Check sheet for the drawn part. Datum: minimum x, y, z corner. Units: mm. A direction names the side the tool comes from. Round coordinates to 2 decimals unless told otherwise and drop trailing zeros. Write each loop counter-clockwise with the first axis right and the second up, starting at its lowest first coordinate (ties: lowest second). Pieces come first, ordered by that corner, then holes. Notation, with made-up numbers: (-24, 29.5) - (1, 29.5) arc R33 ccw to (1, 68.5) - close; hole circle Ø4 at (50, -38.5). An arc over 180 degrees is marked (long way). Answer as a JSON object with one key per item and string values. Group by question number.
1) Mould release check, pull along Z, two halves, no side actions. Record for the marked faces 3, 4 and 5: +Z half, -Z half, draft (parallel to the pull), parting line (faces both ways), or undercut.
2) Go/stop test with flat-tipped pins: pin 1 Ø2 at (x, y) = (8, 6) entering from -Z; pin 2 Ø1 at (x, y) = (10, 2) entering from +Z; pin 3 Ø8 at (y, z) = (8.5, 15.5) entering from +X; pin 4 Ø6.5 at (x, z) = (17.5, 5) entering from +Y. Record where each tip stops, or that it passes through.
3) Thickness scan on line 1 (Z direction, x = 17.5, y = 3.1); line 2 (Z direction, x = 17.5, y = 9.75). Record the ranges inside material, lowest first.
4) Set-up check for the marked faces 1 and 2: record each of +Z, -Z, +X, -X, +Y, -Y from which the full face is reachable in a straight line by a thin tool's end or side.
5) Section check A-A (x = 17.5). Enter the section's corners in (y, z).
6) Section check D-D (x = 12.5). Enter the section's corners in (y, z).
7) Section check B-B (z = 30). Enter the section's corners in (x, y), then the cut area to 3 significant figures.
8) Section check C-C (z = 17.5). Enter the section's corners in (x, y), then the cut area to 3 significant figures.
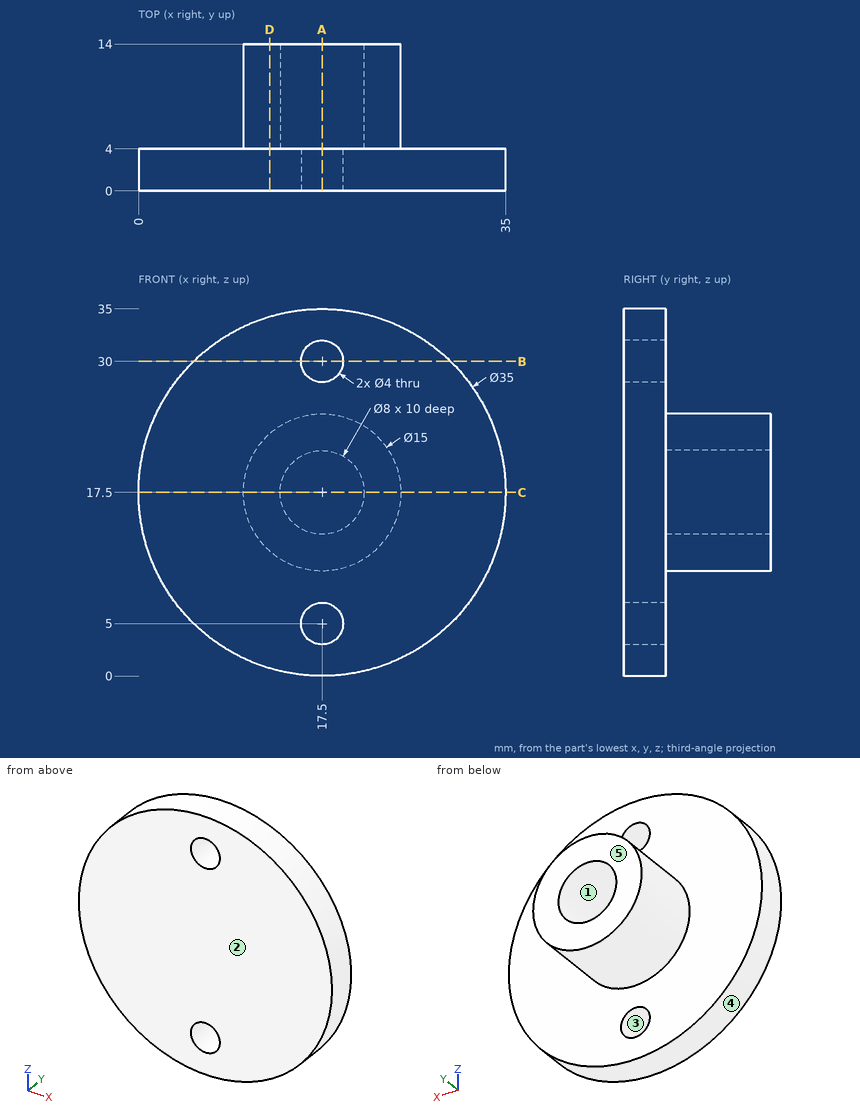
Returned:
{
 "1": {"face 3": "undercut", "face 4": "parting line", "face 5": "draft"},
 "2": {"pin 1": "through", "pin 2": "z = 33.54", "pin 3": "x = 25", "pin 4": "y = 4"},
 "3": {"line 1": "0 to 3, 7 to 28, 32 to 35", "line 2": "10 to 13.5, 21.5 to 25"},
 "4": {"face 1": "+Y", "face 2": "+Z, -Z, +X, -X, -Y"},
 "5": {"outline": "(0, 0) - (4, 0) - (4, 3) - (0, 3) - close; (0, 7) - (4, 7) - (4, 10) - (14, 10) - (14, 13.5) - (4, 13.5) - (4, 21.5) - (14, 21.5) - (14, 25) - (4, 25) - (4, 28) - (0, 28) - close; (0, 32) - (4, 32) - (4, 35) - (0, 35) - close"},
 "6": {"outline": "(0, 0.73) - (4, 0.73) - (4, 11.91) - (14, 11.91) - (14, 23.09) - (4, 23.09) - (4, 34.27) - (0, 34.27) - close"},
 "7": {"outline": "(5.25, 0) - (15.5, 0) - (15.5, 4) - (5.25, 4) - close; (19.5, 0) - (29.75, 0) - (29.75, 4) - (19.5, 4) - close", "area": "82.0 mm2"},
 "8": {"outline": "(0, 0) - (35, 0) - (35, 4) - (25, 4) - (25, 14) - (21.5, 14) - (21.5, 4) - (13.5, 4) - (13.5, 14) - (10, 14) - (10, 4) - (0, 4) - close", "area": "210 mm2"}
}
